Here's how the part is built. I have some questions about the finished solid (model axes, mm). Face numbers are marked on the shaded views. A direction names the side the tool comes from. Coordinates: 2 decimals unless noted, no trailing zeros. Loops run counter-clockwise (first coordinate to the right, second up) from the corner with the lowest first, then second, coordinate; pieces in that order, holes last. Notation, with made-up numbers: (54, 28) -> (101, 28) arc R23 cw to (101, 55) -> close; hole circle Ø3 at (-28.5, 74.25). An arc over 180 degrees is marked (long way). Answer as a JSON object with one key per item and string values. Group by question number.
Q1. I want a section at D-D on x = 19. Write out the boundary of the cut face in (y, z), then the cut area to 3 significant figures.
Q2. I want a section at B-B on z = 16. Write out the boundary of the cut face in (x, y).
Q3. Thinking about a two-plate mould opening in Z: for the marked faces 4, 5, 6 and 7, which applies, released by +Z, released by -Z, zero draft, split by the parting line, or undercut?
Q4. I need wall thicknesses on line 1 (Y direction, x = 0, z = 1.9); line 2 (X direction, y = -15, z = 38.5); line 3 (X direction, y = 18, z = 14.5). Which ranges of each line are inside material? Lowest first, please.
Q5. I want a section at C-C on x = -12. Count the separate pieces of the cut face and the enclosed holes in it, then the cut area to 3 significant figures.
Q6. I'm going to push flat-ended pins straight in: pin 1 (2 mm diameter, centred on x = 10.5, z = 11.5, fed in from -Y); pin 2 (2 mm diameter, centred on x = 13.5, y = -22, fed in from +Z); pin 3 (2.5 mm diameter, centred on x = -12.46, z = 39.4, fed in from -Y). Where does each tip first touch, or does it pass through?
Q7. I want a section at A-A on y = 0. Write out the boundary of the cut face in (x, z).
Q8. On a 3-axis mill with a long thin cutter (end or side, diameter ignored), from which of +Z, -Z, +X, -X, +Y, -Y can I reach the whole of each face in a straight line? I mean the marked faces 1, 2 and 3. Say none if no direction works.
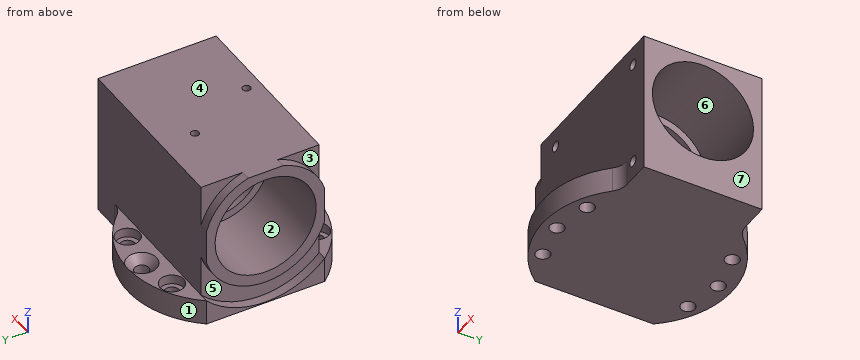
```python
from build123d import *

# Parameters (mm, degrees)
BOSS_EXTRUDE1_DEPTH                                 = 8
CUT_EXTRUDE1_REACH                                  = 5
SKETCH4_W                                           = 55.8
SKETCH4_H                                           = 37.4
BOSS_EXTRUDE2_DEPTH                                 = 37.4
BOSS_EXTRUDE3_DEPTH                                 = 3
CUT_EXTRUDE2_DEPTH                                  = 3
CUT_EXTRUDE3_DEPTH                                  = 3
CSK_FOR_8_FLAT_HEAD_MACHINE_SCREW_100_D             = 4.5
CSK_FOR_8_FLAT_HEAD_MACHINE_SCREW_100_DEPTH         = 8
CSK_FOR_8_FLAT_HEAD_MACHINE_SCREW_100_CSINK_D       = 9.4
CSK_FOR_8_FLAT_HEAD_MACHINE_SCREW_100_CSINK_ANGLE   = 90
F_4_CLEARANCE_HOLE1_D                               = 3.3
F_4_CLEARANCE_HOLE1_DEPTH                           = 6
CBORE_FOR_8_BINDING_HEAD_MACHINE_SCREW1_D           = 4.5
CBORE_FOR_8_BINDING_HEAD_MACHINE_SCREW1_DEPTH       = 8
CBORE_FOR_8_BINDING_HEAD_MACHINE_SCREW1_CBORE_D     = 7.5
CBORE_FOR_8_BINDING_HEAD_MACHINE_SCREW1_CBORE_DEPTH = 3
FILLET1_R                                           = 6.35
M3X0_5_TAPPED_HOLE1_D                               = 2.5
M3X0_5_TAPPED_HOLE1_DEPTH                           = 4
M3X0_5_TAPPED_HOLE1_TIP                             = 0.751075774
FILLET2_R                                           = 6.35
SKETCH_1_R                                          = 16
CUT_EXTRUDE_1_DEPTH                                 = 25.4
SKETCH_2_R                                          = 16
CUT_EXTRUDE_2_DEPTH                                 = 25.4
SKETCH_3_R                                          = 13.55
CUT_EXTRUDE_3_DEPTH                                 = 10


with BuildPart() as part:
    # Sketch1 → Boss-Extrude1 (new body)
    with BuildSketch(Plane.XY.offset(8)):
        with BuildLine():
            Line((-23.45868709, 18.7), (-23.45868709, -18.7))
            ThreePointArc((-23.45868709, -18.7), (0, -30), (23.45868709, -18.7))
            Line((23.45868709, -18.7), (35.34131291, -18.7))
            Line((35.34131291, -18.7), (35.34131291, 18.7))
            Line((35.34131291, 18.7), (23.45868709, 18.7))
            ThreePointArc((23.45868709, 18.7), (0, 30), (-23.45868709, 18.7))
        make_face()
    extrude(amount=-BOSS_EXTRUDE1_DEPTH)

    # Sketch3 → Cut-Extrude1 (cut, up to next)
    with BuildSketch(Plane(origin=(-20.45868709, 0, 0), x_dir=(0, 0, -1), z_dir=(1, 0, 0)), mode=Mode.PRIVATE) as cut_extrude1_sk1:
        with BuildLine():
            Line((-8, 18.7), (-8, -18.7))
            ThreePointArc((-8, -18.7), (-0.254206384, 0), (-8, 18.7))
        make_face()
    cut_extrude1_tool1 = extrude(cut_extrude1_sk1.sketch, amount=-CUT_EXTRUDE1_REACH, mode=Mode.PRIVATE) & part.part
    add(cut_extrude1_tool1.solids().sort_by_distance((-20.458687, 0, 4.859168))[0], mode=Mode.SUBTRACT)

    # Sketch4 → Boss-Extrude2 (add)
    with BuildSketch(Plane.XY.offset(8)):
        with Locations((7.44131291, 0)):
            Rectangle(SKETCH4_W, SKETCH4_H)
    extrude(amount=BOSS_EXTRUDE2_DEPTH)

    # Sketch5 → Boss-Extrude3 (add)
    with BuildSketch(Plane.ZY.offset(20.45868709)):
        with BuildLine():
            Line((21.171890016, 18.7), (45.4, 18.7))
            Line((45.4, 18.7), (45.4, -18.7))
            Line((45.4, -18.7), (21.171890016, -18.7))
            ThreePointArc((21.171890016, -18.7), (7.2, 0), (21.171890016, 18.7))
        make_face()
    extrude(amount=BOSS_EXTRUDE3_DEPTH)

    # Sketch6 → Cut-Extrude2 (cut)
    with BuildSketch(Plane.ZY.offset(23.45868709)):
        with BuildLine():
            Line((45.4, -18.7), (45.4, -5.528109984))
            ThreePointArc((45.4, -5.528109984), (40.488582233, -13.788582233), (32.228109984, -18.7))
            Line((32.228109984, -18.7), (45.4, -18.7))
        make_face()
    extrude(amount=-CUT_EXTRUDE2_DEPTH, mode=Mode.SUBTRACT)

    # Sketch7 → Cut-Extrude3 (cut)
    with BuildSketch(Plane.ZY.offset(23.45868709)):
        with BuildLine():
            Line((45.4, 18.7), (32.228109984, 18.7))
            ThreePointArc((32.228109984, 18.7), (40.488582233, 13.788582233), (45.4, 5.528109984))
            Line((45.4, 5.528109984), (45.4, 18.7))
        make_face()
    extrude(amount=-CUT_EXTRUDE3_DEPTH, mode=Mode.SUBTRACT)

    # Sketch8 → Cut-Revolve1 (revolve, cut)
    with BuildSketch(Plane.XY.offset(26.7)):
        Polygon((-23.45868709, 15.86865), (-23.45868709, 0), (35.34131291, 0), (35.34131291, 15.86865), (9.94131291, 15.86865), (9.94131291, 13.5), (1.94131291, 13.5), (1.94131291, 15.86865), align=None)
    revolve(axis=Axis((-23.45868709, 0, 26.7), (1, 0, 0)), mode=Mode.SUBTRACT)

    # CSK for #8 Flat Head Machine Screw (100)1
    with Locations(Plane.XY.offset(8)):
        with Locations((0, 25.5), (0, -25.5)):
            CounterSinkHole(CSK_FOR_8_FLAT_HEAD_MACHINE_SCREW_100_D / 2, CSK_FOR_8_FLAT_HEAD_MACHINE_SCREW_100_CSINK_D / 2, depth=CSK_FOR_8_FLAT_HEAD_MACHINE_SCREW_100_DEPTH, counter_sink_angle=CSK_FOR_8_FLAT_HEAD_MACHINE_SCREW_100_CSINK_ANGLE)

    # #4 Clearance Hole1
    with Locations(Plane(origin=(0, -18.7, 0), x_dir=(-1, 0, 0), z_dir=(0, -1, 0))):
        with Locations((12.45868709, -39.4), (-29.44131291, -39.4), (-29.44131291, -5.9)):
            Hole(F_4_CLEARANCE_HOLE1_D / 2, depth=F_4_CLEARANCE_HOLE1_DEPTH)

    # CBORE for #8 Binding Head Machine Screw1
    with Locations(Plane.XY.offset(8)):
        with Locations((12, 22.95), (-12, 22.95), (-12, -22.95), (12, -22.95)):
            CounterBoreHole(CBORE_FOR_8_BINDING_HEAD_MACHINE_SCREW1_D / 2, CBORE_FOR_8_BINDING_HEAD_MACHINE_SCREW1_CBORE_D / 2, CBORE_FOR_8_BINDING_HEAD_MACHINE_SCREW1_CBORE_DEPTH, depth=CBORE_FOR_8_BINDING_HEAD_MACHINE_SCREW1_DEPTH)

    # Fillet1
    fillet1_edges = [part.edges().sort_by_distance(p)[0] for p in [
        (23.45868709, 18.7, 4),
    ]]
    fillet(fillet1_edges, radius=FILLET1_R)

    # M3x0.5 Tapped Hole1
    with Locations(Plane(origin=(1.04131291, 8.07366885, 45.4), x_dir=(1, 0, 0), z_dir=(0, 0, 1))):
        with Locations((0, 0), (10.150400418, -22.272670952)):
            Hole(M3X0_5_TAPPED_HOLE1_D / 2, depth=M3X0_5_TAPPED_HOLE1_DEPTH)
            with Locations((0, 0, -(M3X0_5_TAPPED_HOLE1_DEPTH + M3X0_5_TAPPED_HOLE1_TIP / 2))):  # 118° drill point
                Cone(0, M3X0_5_TAPPED_HOLE1_D / 2, M3X0_5_TAPPED_HOLE1_TIP, mode=Mode.SUBTRACT)

    # Fillet2
    fillet2_edges = [part.edges().sort_by_distance(p)[0] for p in [
        (23.45868709, -18.7, 4),
    ]]
    fillet(fillet2_edges, radius=FILLET2_R)

    # 草图1 → 切除-拉伸1 (cut)
    with BuildSketch(Plane(origin=(35.34131291, 0, 0), x_dir=(0, 0, -1), z_dir=(1, 0, 0))):
        with Locations((-26.7, 0)):
            Circle(SKETCH_1_R)
    extrude(amount=-CUT_EXTRUDE_1_DEPTH, mode=Mode.SUBTRACT)

    # 草图2 → 切除-拉伸2 (cut)
    with BuildSketch(Plane.ZY.offset(23.45868709)):
        with Locations((26.7, 0)):
            Circle(SKETCH_2_R)
    extrude(amount=-CUT_EXTRUDE_2_DEPTH, mode=Mode.SUBTRACT)

    # 草图3 → 切除-拉伸3 (cut)
    with BuildSketch(Plane.ZY.offset(-1.94131291)):
        with Locations((26.7, 0)):
            Circle(SKETCH_3_R)
    extrude(amount=-CUT_EXTRUDE_3_DEPTH, mode=Mode.SUBTRACT)


solid = part.part
```
Result set:
{
 "1": {"outline": "(-23.22, 0) -> (23.22, 0) -> (23.22, 8) -> (18.7, 8) -> (18.7, 45.4) -> (-18.7, 45.4) -> (-18.7, 8) -> (-23.22, 8) -> close; hole circle Ø32 at (0, 26.7)", "area": "966 mm²"},
 "2": {"outline": "(-23.46, -16.3) -> (-20.46, -16.3) -> (-20.46, -18.7) -> (35.34, -18.7) -> (35.34, -11.9) -> (9.94, -11.9) -> (9.94, -8.31) -> (1.94, -8.31) -> (1.94, -11.9) -> (-23.46, -11.9) -> close; (-23.46, 11.9) -> (1.94, 11.9) -> (1.94, 8.31) -> (9.94, 8.31) -> (9.94, 11.9) -> (35.34, 11.9) -> (35.34, 18.7) -> (-20.46, 18.7) -> (-20.46, 16.3) -> (-23.46, 16.3) -> close"},
 "3": {"face 4": "released by +Z", "face 5": "undercut", "face 6": "undercut", "face 7": "zero draft"},
 "4": {"line 1": "y = -30 to -27.75, -23.25 to 23.25, 27.75 to 30", "line 2": "x = -23.46 to -13.84, -11.08 to 28.06, 30.82 to 35.34", "line 3": "x = -20.46 to 35.34"},
 "5": {"separate pieces": "3", "enclosed holes": "1", "area": "925 mm²"},
 "6": {"pin 1": "stops at y = -18.7", "pin 2": "stops at z = 5", "pin 3": "stops at y = -12.7"},
 "7": {"outline": "(-23.46, 0) -> (35.34, 0) -> (35.34, 10.7) -> (9.94, 10.7) -> (9.94, 13.15) -> (1.94, 13.15) -> (1.94, 10.7) -> (-23.46, 10.7) -> (-23.46, 7.2) -> (-20.46, 7.2) -> (-20.46, 0.25) -> (-23.46, 0.25) -> close; (-23.46, 42.7) -> (1.94, 42.7) -> (1.94, 40.25) -> (9.94, 40.25) -> (9.94, 42.7) -> (35.34, 42.7) -> (35.34, 45.4) -> (-23.46, 45.4) -> close"},
 "8": {"face 1": "+Z, -Z, +Y", "face 2": "-X", "face 3": "+Z, -X, -Y"}
}
